Check sheet for the modelled part. Datum: model origin and axes. Units: mm. Round coordinates to 2 decimals unless told otherwise and drop trailing zeros. Write each loop counter-clockwise with the first axis right and the second up, starting at its lowest first coordinate (ties: lowest second). Pieces come first, ordered by that corner, then holes.
from build123d import *

# Parameters (mm, degrees)
SKETCH2_W           = 3.05
SKETCH2_H           = 2.25
SKETCH2_W_2         = 2.2
SKETCH2_H_2         = 2
SKETCH2_W_3         = 1.5
SKETCH2_H_3         = 2.2
BOSS_EXTRUDE1_DEPTH = 1000
FILLET1_R           = 0.5
FILLET2_R           = 0.5


with BuildPart() as part:
    # Sketch2 → Boss-Extrude1 (new body)
    with BuildSketch(Plane.XY):
        with Locations((0.108353761, 4.001842427)):
            Rectangle(SKETCH2_W, SKETCH2_H)
        Polygon((-1.416646239, -1.873157573), (-1.416646239, 2.876842427), (-4.466646239, 2.876842427), (-4.466646239, 0.126842427), (-4.466646239, -1.873157573), (-4.216646239, -1.873157573), (-2.716646239, -1.873157573), align=None)
        Polygon((1.633353761, 2.876842427), (-1.416646239, 2.876842427), (-1.416646239, -1.873157573), (-0.116646239, -1.873157573), (1.383353761, -1.873157573), (1.633353761, -1.873157573), (1.633353761, 0.126842427), align=None)
        with Locations((-2.941646239, 4.001842427)):
            Rectangle(SKETCH2_W, SKETCH2_H)
        with Locations((2.733353761, -0.873157573)):
            Rectangle(SKETCH2_W_2, SKETCH2_H_2)
        with Locations((0.633353761, -2.973157573)):
            Rectangle(SKETCH2_W_3, SKETCH2_H_3)
        with Locations((-3.466646239, -2.973157573)):
            Rectangle(SKETCH2_W_3, SKETCH2_H_3)
        with Locations((-5.566646239, -0.873157573)):
            Rectangle(SKETCH2_W_2, SKETCH2_H_2)
    extrude(amount=BOSS_EXTRUDE1_DEPTH)

    # Fillet1
    fillet1_edges = [part.edges().sort_by_distance(p)[0] for p in [
        (3.833353761, 0.126842427, 500),
        (3.833353761, -1.873157573, 500),
        (-6.666646239, -1.873157573, 500),
        (-6.666646239, 0.126842427, 500),
    ]]
    fillet(fillet1_edges, radius=FILLET1_R)

    # Fillet2
    fillet2_edges = [part.edges().sort_by_distance(p)[0] for p in [
        (1.383353761, -4.073157573, 500),
        (-0.116646239, -4.073157573, 500),
        (-2.716646239, -4.073157573, 500),
        (-4.216646239, -4.073157573, 500),
    ]]
    fillet(fillet2_edges, radius=FILLET2_R)


solid = part.part
1. Scan lines: line 1 along X through (y, z) = (-2, 501); line 2 along X through (y, z) = (-1.5, 398); line 3 along Y through (x, z) = (-0.25, 732.5). Record each from-to range of solid material in increasing order.
2. Sectioned sample at B-B, the plane y = 2.25. Enter the section's corners in (x, z), plus the area to 3 significant figures.
3. Go/stop test with flat-tipped pins: pin 1 (0.8 mm diameter, centred on y = -2.5, z = 581.5, fed in from +X); pin 2 (1.4 mm diameter, centred on x = 2.5, z = 608.5, fed in from +Y); pin 3 (0.8 mm diameter, centred on y = -2.5, z = 349, fed in from -X). Record where each tip stops, or that it passes through.
4. Sectioned sample at A-A, the plane z = 723. Enter the section's corners in (x, y), plus the area to 3 significant figures.
Computed values:
1. line 1: x = -4.22 to -2.72, -0.12 to 1.38
1. line 2: x = -6.65 to 3.82
1. line 3: y = -1.87 to 5.13
2. outline: (-4.47, 0) - (1.63, 0) - (1.63, 1000) - (-4.47, 1000) - close
2. area: 6,100 mm2
3. pin 1: stops at x = 1.38
3. pin 2: stops at y = 0.13
3. pin 3: stops at x = -4.22
4. outline: (-6.67, -1.37) arc R0.5 ccw to (-6.17, -1.87) - (-4.22, -1.87) - (-4.22, -3.57) arc R0.5 ccw to (-3.72, -4.07) - (-3.22, -4.07) arc R0.5 ccw to (-2.72, -3.57) - (-2.72, -1.87) - (-0.12, -1.87) - (-0.12, -3.57) arc R0.5 ccw to (0.38, -4.07) - (0.88, -4.07) arc R0.5 ccw to (1.38, -3.57) - (1.38, -1.87) - (3.33, -1.87) arc R0.5 ccw to (3.83, -1.37) - (3.83, -0.37) arc R0.5 ccw to (3.33, 0.13) - (1.63, 0.13) - (1.63, 5.13) - (-4.47, 5.13) - (-4.47, 0.13) - (-6.17, 0.13) arc R0.5 ccw to (-6.67, -0.37) - close
4. area: 57.7 mm2
